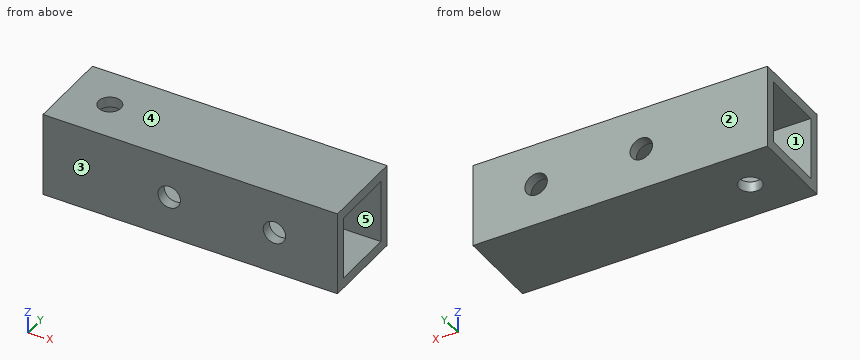
from build123d import *

# Parameters (mm, degrees)
SKETCH_1_W          = 12
SKETCH_1_H          = 12
SKETCH_1_W_2        = 9
SKETCH_1_H_2        = 9
EXTRUDE_1_DEPTH     = 21
SKETCH_4_R          = 1.6
CUT_EXTRUDE_3_DEPTH = 13
SKETCH_5_R          = 1.6
CUT_EXTRUDE_4_DEPTH = 13


with BuildPart() as part:
    # ｽｹｯﾁ1 → ﾎﾞｽ - 押し出し1 (new body, symmetric)
    with BuildSketch(Plane(origin=(0, 0, 0), x_dir=(0, 0, -1), z_dir=(1, 0, 0))):
        Rectangle(SKETCH_1_W, SKETCH_1_H)
        Rectangle(SKETCH_1_W_2, SKETCH_1_H_2, mode=Mode.SUBTRACT)
    extrude(amount=EXTRUDE_1_DEPTH, both=True)

    # ｽｹｯﾁ4 → ｶｯﾄ - 押し出し3 (cut, through all)
    with BuildSketch(Plane(origin=(0, 6, 0), x_dir=(1, 0, 0), z_dir=(0, 1, 0))):
        with Locations((-3, 0)):
            Circle(SKETCH_4_R)
        with Locations((12, 0)):
            Circle(SKETCH_4_R)
    extrude(amount=-CUT_EXTRUDE_3_DEPTH, mode=Mode.SUBTRACT)

    # ｽｹｯﾁ5 → ｶｯﾄ - 押し出し4 (cut, through all)
    with BuildSketch(Plane.XY.offset(6)):
        with Locations((-15, 0)):
            Circle(SKETCH_5_R)
    extrude(amount=-CUT_EXTRUDE_4_DEPTH, mode=Mode.SUBTRACT)


solid = part.part
Source: CAD feature listing. Evaluate the final solid. Frame: model axes, mm. Face numbers are marked on the shaded views. A direction names the side the tool comes from. Coordinates: 2 decimals unless noted, no trailing zeros. Loops run counter-clockwise (first coordinate to the right, second up) from the corner with the lowest first, then second, coordinate; pieces in that order, holes last. Notation, with made-up numbers: (23, 31) - (45, 31) arc R21 cw to (45, 44) - close; hole circle Ø1 at (-1.5, -1). An arc over 180 degrees is marked (long way). One line per question, with ' | ' between items.
1) Section C-C, the plane x = -7.5. Return loops of the section in (y, z).
Report:
outline: (-6, -6) - (6, -6) - (6, 6) - (-6, 6) - close; hole (-4.5, -4.5) - (4.5, -4.5) - (4.5, 4.5) - (-4.5, 4.5) - close
2) First-contact query: P1, Ø3, axis at x = 12, z = 0, coming from the -Y side. Flat tip, straight axial feed; report the tip coordinate or a pass-through.
Report:
P1: passes through
3) Section D-D, the plane z = 0. Return loops of the section in (x, y).
Report:
outline: (-21, -6) - (-4.6, -6) - (-4.6, -4.5) - (-21, -4.5) - close; (-21, 4.5) - (-4.6, 4.5) - (-4.6, 6) - (-21, 6) - close; (-1.4, -6) - (10.4, -6) - (10.4, -4.5) - (-1.4, -4.5) - close; (-1.4, 4.5) - (10.4, 4.5) - (10.4, 6) - (-1.4, 6) - close; (13.6, -6) - (21, -6) - (21, -4.5) - (13.6, -4.5) - close; (13.6, 4.5) - (21, 4.5) - (21, 6) - (13.6, 6) - close
4) Section A-A, the plane z = -2.75. Return loops of the section in (x, y).
Report:
outline: (-21, -6) - (21, -6) - (21, -4.5) - (-21, -4.5) - close; (-21, 4.5) - (21, 4.5) - (21, 6) - (-21, 6) - close
5) Line query: line 1 along X through (y, z) = (-5, 0); line 2 along Z through (x, y) = (-3, -4.95); line 3 along Y through (x, z) = (7, -2). Output: solid intervals per line, ascending.
Report:
line 1: x = -21 to -4.6, -1.4 to 10.4, 13.6 to 21 | line 2: z = -6 to -1.6, 1.6 to 6 | line 3: y = -6 to -4.5, 4.5 to 6
6) Pull-direction query (Z, two-part tool) for the marked faces 3, 4 and 5; classes: released by +Z, released by -Z, zero draft, split by the parting line, or undercut.
Report:
face 3: zero draft | face 4: released by +Z | face 5: undercut
7) Set-up query: the marked faces 1 and 2. Return all of +Z, -Z, +X, -X, +Y, -Y with unobstructed straight access to the full face (end or side cutting, diameter ignored); none if empty.
Report:
face 1: +X, -X | face 2: +Z, -Z, +X, -X, +Y
8) Section B-B, the plane y = 0. Return loops of the section in (x, z).
Report:
outline: (-21, -6) - (-16.6, -6) - (-16.6, -4.5) - (-21, -4.5) - close; (-21, 4.5) - (-16.6, 4.5) - (-16.6, 6) - (-21, 6) - close; (-13.4, -6) - (21, -6) - (21, -4.5) - (-13.4, -4.5) - close; (-13.4, 4.5) - (21, 4.5) - (21, 6) - (-13.4, 6) - close
